Read the model definition and answer for the solid it produces. Units are mm, in the model's axes. Face numbers are marked on the shaded views. Round coordinates to 2 decimals unless told otherwise and drop trailing zeros. Loops run counter-clockwise (first coordinate to the right, second up) from the corner with the lowest first, then second, coordinate; pieces in that order, holes last. Notation, with made-up numbers: (62.25, 89) -> (72.25, 89) arc R18 ccw to (72.25, 104) -> close; hole circle Ø1 at (62.25, 50). An arc over 180 degrees is marked (long way). Put each result on its own line as item: value.
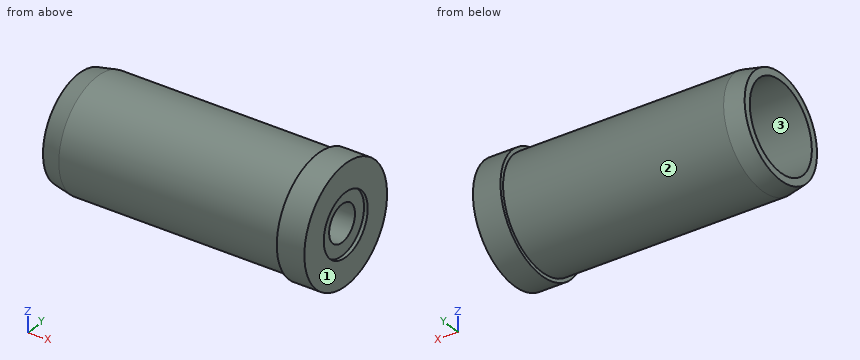
from build123d import *


with BuildPart() as part:
    # Esquisse1 → Révolution1 (revolve)
    with BuildSketch(Plane.XY, mode=Mode.PRIVATE) as r_volution1_sk:
        Polygon((175.54977417, 10), (175.54977417, 17), (177.54977417, 17), (177.54977417, 32), (162.54977417, 32), (162.54977417, 30), (42.566441994, 30), (32.54977417, 28), (32.54977417, 24), (162.54977417, 24), (162.54977417, 10), align=None)
    revolve(r_volution1_sk.sketch.rotate(Axis((32.54977417, 0, 0), (1, 0, 0)), 270), axis=Axis((32.54977417, 0, 0), (1, 0, 0)))


solid = part.part
Item 1: The part is cut by section A-A (z = 0). Determine the outline of the cut face in (x, y), then the cut area to 3 significant figures.
Derived:
outline: (32.55, -28) -> (42.57, -30) -> (162.55, -30) -> (162.55, -32) -> (177.55, -32) -> (177.55, -17) -> (175.55, -17) -> (175.55, -10) -> (162.55, -10) -> (162.55, -24) -> (32.55, -24) -> close; (32.55, 24) -> (162.55, 24) -> (162.55, 10) -> (175.55, 10) -> (175.55, 17) -> (177.55, 17) -> (177.55, 32) -> (162.55, 32) -> (162.55, 30) -> (42.57, 30) -> (32.55, 28) -> close
area: 2,170 mm^2
Item 2: Find the intervals of material crossed by line 1 along Y through (x, z) = (171.5, 0); line 2 along Y through (x, z) = (176, 0); line 3 along X through (y, z) = (8.5, 9.5), in increasing order.
Derived:
line 1: y = -32 to -10, 10 to 32
line 2: y = -32 to -17, 17 to 32
line 3: x = 162.55 to 175.55
Item 3: For a pull along Z with two mould halves and no side action, classify the marked faces 1, 2 and 3 as pulls with the +Z half, pulls with the -Z half, needs draft (parallel to the pull), parting line crosses it, or undercut.
Derived:
face 1: needs draft
face 2: parting line crosses it
face 3: undercut
Item 4: The part is cut by section C-C (x = 63.5). Determine the outline of the cut face in (y, z), then the cut area to 3 significant figures.
Derived:
outline: circle Ø60 at (0, 0); hole circle Ø48 at (0, 0)
area: 1,020 mm^2
Item 5: Flat-ended cylindrical pins translate along their axes: pin 1 Ø6 at (x, z) = (79, 25.5) entering from -Y; pin 2 Ø8 at (x, z) = (87, -14) entering from -Y; pin 3 Ø2 at (x, z) = (62, 12.5) entering from -Y. Find the tip coordinate at first contact, or state that the pin passes through.
Derived:
pin 1: stops at y = -19.84
pin 2: stops at y = -28.28
pin 3: stops at y = -27.71
